Study the drawing (mm; zero at the part's minimum x, y, z) and answer. A direction names the side the tool comes from. Round coordinates to 2 decimals unless told otherwise and drop trailing zeros. Write each loop counter-clockwise with the first axis right and the second up, starting at its lowest first coordinate (ties: lowest second). Pieces come first, ordered by that corner, then holes. Notation, with made-up numbers: (-36, -21) -> (-16, -21) arc R6 cw to (-16, -16) -> close; hole circle Ø2 at (-23.5, 26.25). An arc over 180 degrees is marked (long way). Write each question's results on one line, items separated by ' | '. Start each with the question number.
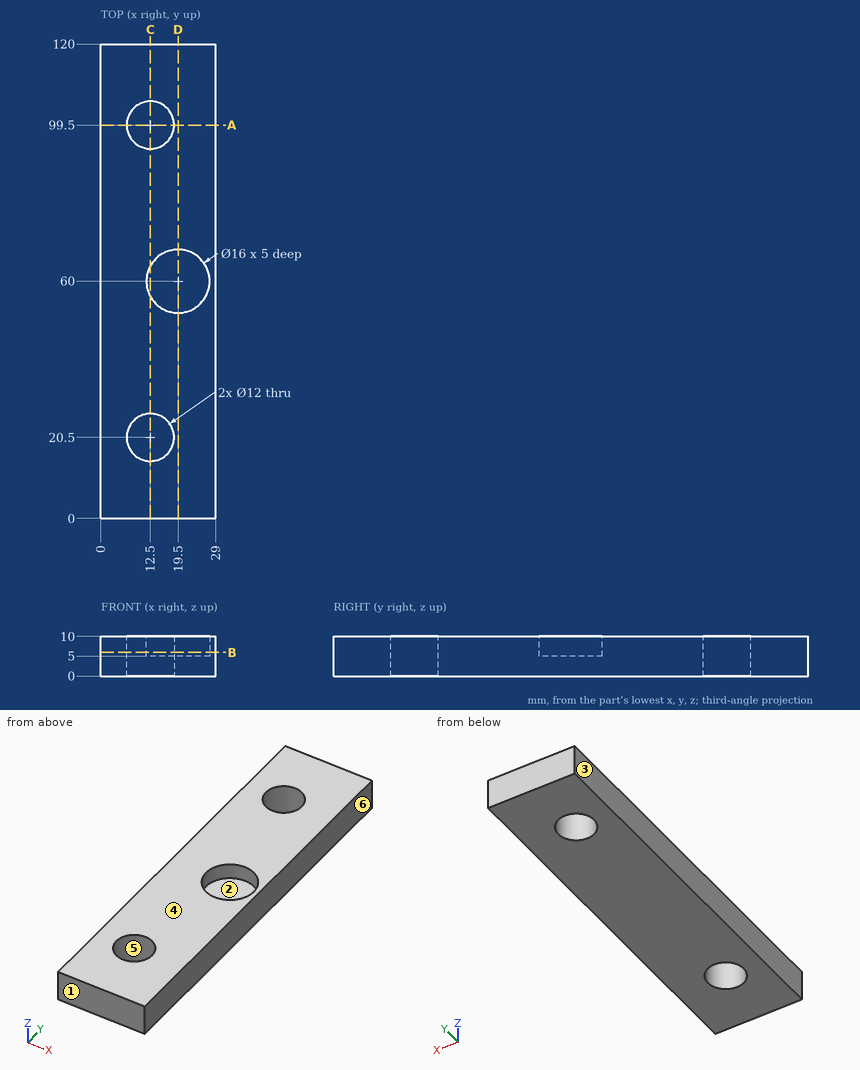
Q1. For the marked faces 1 and 2, determine the directions among +Z, -Z, +X, -X, +Y, -Y from which every point of the face is accessible in a straight line to the end or side of a thin tool.
Q2. The part is cut by section C-C, the plane x = 12.5. Write down the section's boundary in (y, z).
Q3. Find the intervals of material crossed by line 1 (Y direction, x = 11.25, z = 5.75); line 2 (Y direction, x = 12.5, z = 2.5); line 3 (Y direction, x = 19.5, z = 8.85), in increasing order.
Q4. Determine the mould class of the marked faces 3, 4, 5 and 6 for opening direction X: pulls with the +X half, pulls with the -X half, needs draft (parallel to the pull), parting line crosses it, or undercut.
Q5. The part is cut by section A-A, the plane y = 99.5. Write down the section's boundary in (x, z), then the cut area to 3 significant figures.
Q6. Each of these flat-tipped pins is pushed along its axis until it touches: pin 1 (7 mm diameter, centred on x = 12.5, y = 20.5, fed in from -Z); pin 2 (2 mm diameter, centred on x = 21, y = 12.5, fed in from -Z). Where does it stop, or does it pass through?
Q7. The part is cut by section B-B, the plane z = 6. Write down the section's boundary in (x, y), then the cut area to 3 significant figures.
Q8. The part is cut by section D-D, the plane x = 19.5. Write down the section's boundary in (y, z).
Answers follow:
1) face 1: +Z, -Z, +X, -X, -Y | face 2: +Z
2) outline: (0, 0) -> (14.5, 0) -> (14.5, 10) -> (0, 10) -> close; (26.5, 0) -> (93.5, 0) -> (93.5, 10) -> (63.87, 10) -> (63.87, 5) -> (56.13, 5) -> (56.13, 10) -> (26.5, 10) -> close; (105.5, 0) -> (120, 0) -> (120, 10) -> (105.5, 10) -> close
3) line 1: 0 to 14.63, 26.37 to 93.63, 105.37 to 120 | line 2: 0 to 14.5, 26.5 to 93.5, 105.5 to 120 | line 3: 0 to 52, 68 to 120
4) face 3: pulls with the -X half | face 4: needs draft | face 5: undercut | face 6: pulls with the +X half
5) outline: (0, 0) -> (6.5, 0) -> (6.5, 10) -> (0, 10) -> close; (18.5, 0) -> (29, 0) -> (29, 10) -> (18.5, 10) -> close | area: 170 mm^2
6) pin 1: through | pin 2: z = 0
7) outline: (0, 0) -> (29, 0) -> (29, 120) -> (0, 120) -> close; hole circle Ø12 at (12.5, 20.5); hole circle Ø12 at (12.5, 99.5); hole circle Ø16 at (19.5, 60) | area: 3,050 mm^2
8) outline: (0, 0) -> (120, 0) -> (120, 10) -> (68, 10) -> (68, 5) -> (52, 5) -> (52, 10) -> (0, 10) -> close
